```python
from build123d import *

# Parameters (mm, degrees)
F0_W     = 55.39994
F0_H     = 50.40122
F0_W_2   = 29.99994
F0_H_2   = 25.00122
F1_DEPTH = 1.5875
F2_W     = 55.39994
F2_H     = 3.175
F3_DEPTH = 52.96154


with BuildPart() as f1:
    # F0 (on Front) → F1 (new body, symmetric)
    with BuildSketch(Plane.XZ):
        Rectangle(F0_W, F0_H)
        Rectangle(F0_W_2, F0_H_2, mode=Mode.SUBTRACT)
    extrude(amount=F1_DEPTH, both=True)

    # F2 (on face) → F3 (join)
    with BuildSketch(Plane.XZ.offset(1.5875)):
        with Locations((0, 23.61311)):
            Rectangle(F2_W, F2_H)
    extrude(amount=F3_DEPTH)


solid = f1.part
```
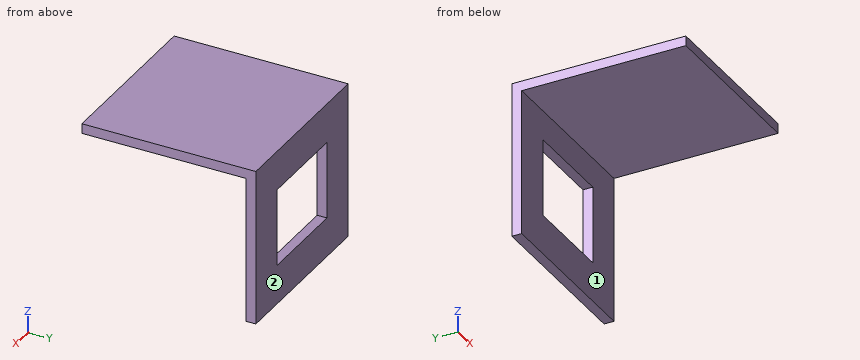
Geometry check sheet. Reference: the model listing, model coordinates, mm. Face numbers are marked on the shaded views. A direction names the side the tool comes from. Coordinates: 2 decimals unless noted, no trailing zeros. Loops run counter-clockwise (first coordinate to the right, second up) from the corner with the lowest first, then second, coordinate; pieces in that order, holes last.
Item 1: Sectioned sample at B-B, the plane x = 1.5. Record the boundary of the cut face in (y, z).
Item 2: Thickness scan on line 1 (Z direction, x = -17, y = -45); line 2 (Y direction, x = 22.5, z = 0.5). Record the ranges inside material, lowest first.
Item 3: Sectioned sample at A-A, the plane z = 8. Record the boundary of the cut face in (x, y), then the cut area to 3 significant figures.
Item 4: Sectioned sample at D-D, the plane z = -17. Record the boundary of the cut face in (x, y).
Item 5: Go/stop test with flat-tipped pins: pin 1 Ø14 at (x, z) = (3.5, 2.5) entering from -Y; pin 2 Ø5 at (x, z) = (11.5, 11.5) entering from -Y; pin 3 Ø2 at (x, y) = (12, -14) entering from -Z. Record where each tip stops, or that it passes through.
Item 6: Access from +Z, -Z, +X, -X, +Y, -Y to the whole of each face (thin tool, end or side, straight path). Record for the marked faces 1 and 2.
Item 7: Sectioned sample at C-C, the plane x = -16. Record the boundary of the cut face in (y, z), then the cut area to 3 significant figures.
Check result:
1. outline: (-54.55, 22.03) - (-1.59, 22.03) - (-1.59, 12.5) - (1.59, 12.5) - (1.59, 25.2) - (-54.55, 25.2) - close; (-1.59, -25.2) - (1.59, -25.2) - (1.59, -12.5) - (-1.59, -12.5) - close
2. line 1: z = 22.03 to 25.2
2. line 2: y = -1.59 to 1.59
3. outline: (-27.7, -1.59) - (-15, -1.59) - (-15, 1.59) - (-27.7, 1.59) - close; (15, -1.59) - (27.7, -1.59) - (27.7, 1.59) - (15, 1.59) - close
3. area: 80.6 mm2
4. outline: (-27.7, -1.59) - (27.7, -1.59) - (27.7, 1.59) - (-27.7, 1.59) - close
5. pin 1: passes through
5. pin 2: stops at y = -1.59
5. pin 3: stops at z = 22.03
6. face 1: -Z, +X, -X, -Y
6. face 2: +Z, -Z, +X, -X, +Y
7. outline: (-54.55, 22.03) - (-1.59, 22.03) - (-1.59, -25.2) - (1.59, -25.2) - (1.59, 25.2) - (-54.55, 25.2) - close
7. area: 328 mm2
